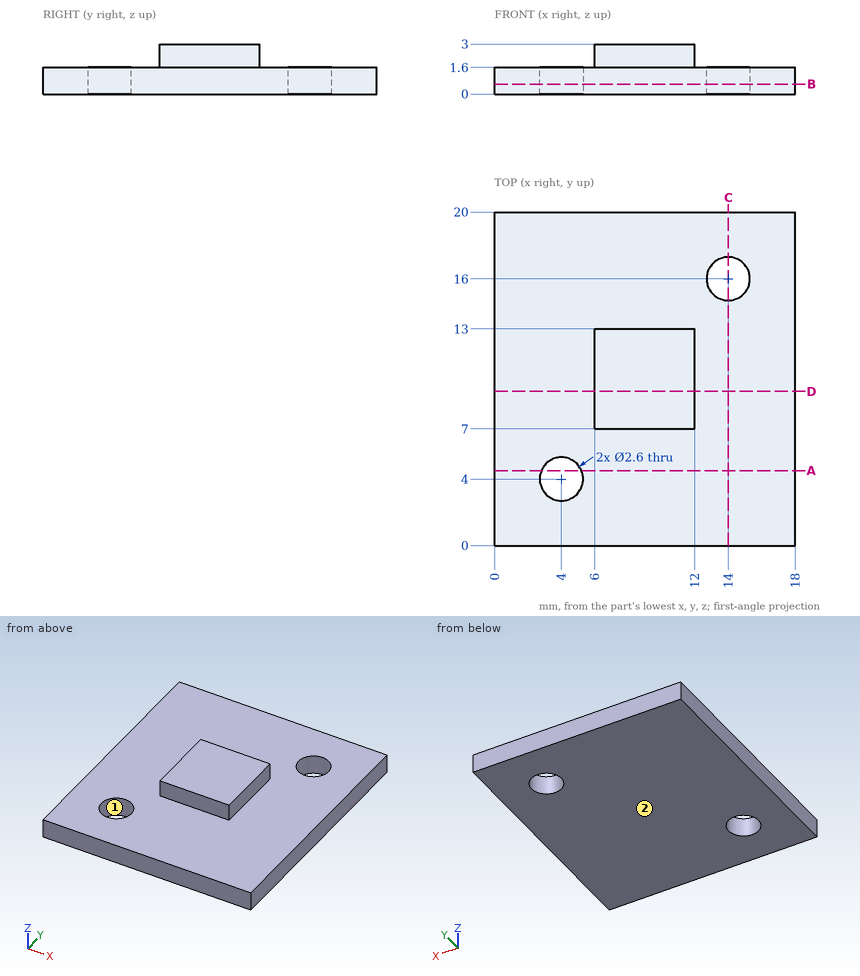
Study the drawing (mm; zero at the part's minimum x, y, z) and answer. Coordinates: 2 decimals unless noted, no trailing zeros. Write each loop counter-clockwise with the first axis right and the second up, starting at its lowest first coordinate (ties: lowest second). Pieces come first, ordered by that corner, then holes. Notation, with made-up numbers: (-38, 3) -> (15, 3) arc R35 cw to (15, 38) -> close; hole circle Ø1 at (-22, 84). An arc over 180 degrees is marked (long way). Write each question's results on one line, items separated by ' | '. Start each with the question number.
1) For a pull along Y with two mould halves and no side action, classify the marked faces 1 and 2 as +Y half, -Y half, draft (parallel to the pull), parting line (faces both ways), or undercut.
2) A cutting plane is placed at B-B (z = 0.6). Determine the outline of the cut face in (x, y), then the cut area to 3 significant figures.
3) A cutting plane is placed at A-A (y = 4.5). Determine the outline of the cut face in (x, z).
4) Straight lines are drawn through the part: probe 1 along Y at (x, z) = (4, 0.55); probe 2 along Y at (x, z) = (14, 0.9); probe 3 along X at (y, z) = (16, 1). For each, find the intervals that lie inside material, in ascending order.
5) A cutting plane is placed at C-C (x = 14). Determine the outline of the cut face in (y, z).
6) A cutting plane is placed at D-D (y = 9.25). Determine the outline of the cut face in (x, z), then the cut area to 3 significant figures.
7) Flat-ended cylindrical pins translate along their axes: pin 1 Ø4 at (x, y) = (4, 4) entering from +Z; pin 2 Ø1.5 at (y, z) = (10.5, 2.5) entering from -X; pin 3 Ø1.5 at (y, z) = (10, 2.5) entering from +X. Find the tip coordinate at first contact, or state that the pin passes through.
Values follow:
1) face 1: undercut | face 2: draft
2) outline: (0, 0) -> (18, 0) -> (18, 20) -> (0, 20) -> close; hole circle Ø2.6 at (4, 4); hole circle Ø2.6 at (14, 16) | area: 349 mm²
3) outline: (0, 0) -> (2.8, 0) -> (2.8, 1.6) -> (0, 1.6) -> close; (5.2, 0) -> (18, 0) -> (18, 1.6) -> (5.2, 1.6) -> close
4) probe 1: 0 to 2.7, 5.3 to 20 | probe 2: 0 to 14.7, 17.3 to 20 | probe 3: 0 to 12.7, 15.3 to 18
5) outline: (0, 0) -> (14.7, 0) -> (14.7, 1.6) -> (0, 1.6) -> close; (17.3, 0) -> (20, 0) -> (20, 1.6) -> (17.3, 1.6) -> close
6) outline: (0, 0) -> (18, 0) -> (18, 1.6) -> (12, 1.6) -> (12, 3) -> (6, 3) -> (6, 1.6) -> (0, 1.6) -> close | area: 37.2 mm²
7) pin 1: z = 1.6 | pin 2: x = 6 | pin 3: x = 12
